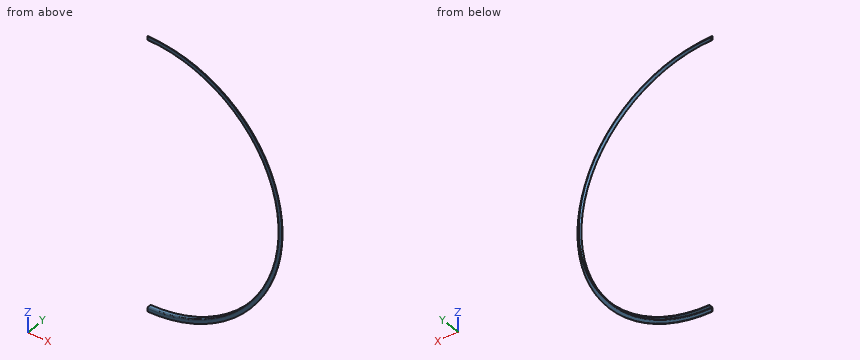
from build123d import *

# Parameters (mm, degrees)
BASE_FLANGE1_DEPTH   = 4
EDGE_FLANGE1_ANGLE   = 180
EDGE_FLANGE1_2_ANGLE = 180


# Read off the part's stored shape, not the designer's step: Edge-Flange1
# Sheet-metal steps are written as plain solids
with BuildPart() as part:
    # Sketch1 → Base-Flange1 (new body)
    with BuildSketch(Plane(origin=(0, 0, 0), x_dir=(1, 0, 0), z_dir=(0, 1, 0))):
        with BuildLine():
            Line((0, 1290), (0, 1250))
            ThreePointArc((0, 1250), (1250, 0), (0, -1250))
            Line((0, -1250), (0, -1290))
            ThreePointArc((0, -1290), (1290, 0), (0, 1290))
        make_face()
    extrude(amount=-BASE_FLANGE1_DEPTH)

    # Edge-Flange1 outline → Edge-Flange1 (revolve, cut)
    with BuildSketch(Plane.ZY):
        with BuildLine():
            Line((1252, 0), (1250, 0))
            Line((1250, 0), (1250, -4))
            Line((1250, -4), (1260, -4))
            ThreePointArc((1260, -4), (1255.527864045, -2.94427191), (1252, 0))
        make_face()
    revolve(axis=Axis((0, 0, 0), (0, 1, 0)), revolution_arc=EDGE_FLANGE1_ANGLE, mode=Mode.SUBTRACT)

    # Edge-Flange1 2 outline → Edge-Flange1 2 (revolve)
    with BuildSketch(Plane.ZY):
        with BuildLine():
            Line((1254, 36), (1250, 36))
            Line((1250, 36), (1250, 6))
            ThreePointArc((1250, 6), (1250.513167019, 2.83772234), (1252, 0))
            Line((1252, 0), (1260, 0))
            ThreePointArc((1260, 0), (1255.757359313, 1.757359313), (1254, 6))
            Line((1254, 6), (1254, 36))
        make_face()
    revolve(axis=Axis((0, 0, 0), (0, 1, 0)), revolution_arc=EDGE_FLANGE1_2_ANGLE)


solid = part.part
Here's how the part is built. I have some questions about the finished solid (model axes, mm). Give positions to 0.01 mm unless a question says otherwise; leave off trailing zeros. Loops run counter-clockwise (first coordinate to the right, second up) from the corner with the lowest first, then second, coordinate; pieces in that order, holes last. Notation, with made-up numbers: (-40, -26) -> (14, -26) arc R29 cw to (14, -2) -> close; hole circle Ø6 at (-8, 32). An arc over 180 degrees is marked (long way). Answer as a JSON object with one key per item and string values. Group by question number.
Item 1: Imagine slicing it at A-A on y = 21. Write out the boundary of the cut face in (x, z), then the cut area to 3 significant figures.
Item 2: Will these pins go through, and if not, where does the flat tip stop? pin 1 (8 mm diameter, centred on x = 940, y = 30.5, fed in from +Z); pin 2 (6 mm diameter, centred on y = 5.5, z = 695.5, fed in from -X); pin 3 (5 mm diameter, centred on x = 349.5, y = 16, fed in from -Z).
Item 3: I need wall thicknesses on L1, parallel to Z at x = 639, y = 4; L2, parallel to Z at x = 375, y = 18.5; L3, parallel to Y at x = 976.5, z = -842. Which ranges of each line are inside material? Lowest first, please.
Answer list:
{
 "1": {"outline": "(0, -1254) arc R1254 ccw to (0, 1254) -> (0, 1250) arc R1250 cw to (0, -1250) -> close", "area": "15,700 mm2"},
 "2": {"pin 1": "stops at z = 834.52", "pin 2": "stops at x = 1036.64", "pin 3": "stops at z = -1205.03"},
 "3": {"L1": "z = -1079.38 to -1074.56, 1074.56 to 1079.38", "L2": "z = -1196.62 to -1192.42, 1192.42 to 1196.62", "L3": "y = -4 to 0"}
}
